```python
from build123d import *

# Parameters (mm, degrees)
BOSS_EXTRUDE1_DEPTH = 5.842
SKETCH2_R           = 3.175
CUT_EXTRUDE1_DEPTH  = 50.679572542


with BuildPart() as part:
    # Sketch1 → Boss-Extrude1 (new body)
    with BuildSketch(Plane(origin=(0, 0, 0), x_dir=(1, 0, 0), z_dir=(0, 1, 0))):
        Polygon((38.1, -25.5), (31.725545431, -25.5), (31.725545431, -31.342), (19.025545431, -31.342), (19.025545431, -25.5), (14.4526, -25.5), (14.4526, -19.15), (15.748, -19.15), (15.748, -15.975), (14.4526, -15.975), (14.4526, -11.403), (10.9474, -11.403), (10.9474, -15.975), (9.652, -15.975), (9.652, -19.15), (10.9474, -19.15), (10.9474, -25.5), (6.325545431, -25.5), (6.325545431, -31.342), (-6.374454569, -31.342), (-6.374454569, -25.5), (-10.996309138, -25.5), (-10.996309138, -19.15), (-9.700909138, -19.15), (-9.700909138, -15.975), (-10.996309138, -15.975), (-10.996309138, -11.403), (-14.501509138, -11.403), (-14.501509138, -15.975), (-15.796909138, -15.975), (-15.796909138, -19.15), (-14.501509138, -19.15), (-14.501509138, -25.5), (-19.074454569, -25.5), (-19.074454569, -31.342), (-31.774454569, -31.342), (-31.774454569, -25.5), (-38.1, -25.5), (-38.1, 25.5), (-31.774454569, 25.5), (-31.774454569, 31.342), (-19.074454569, 31.342), (-19.074454569, 25.5), (-14.501509138, 25.5), (-14.501509138, 19.15), (-15.796909138, 19.15), (-15.796909138, 15.975), (-14.501509138, 15.975), (-14.501509138, 11.403), (-10.996309138, 11.403), (-10.996309138, 15.975), (-9.700909138, 15.975), (-9.700909138, 19.15), (-10.996309138, 19.15), (-10.996309138, 25.5), (-6.374454569, 25.5), (-6.374454569, 31.342), (6.325545431, 31.342), (6.325545431, 25.5), (10.9474, 25.5), (10.9474, 19.15), (9.652, 19.15), (9.652, 15.975), (10.9474, 15.975), (10.9474, 11.403), (14.4526, 11.403), (14.4526, 15.975), (15.748, 15.975), (15.748, 19.15), (14.4526, 19.15), (14.4526, 25.5), (19.025545431, 25.5), (19.025545431, 31.342), (31.725545431, 31.342), (31.725545431, 25.5), (38.1, 25.5), align=None)
    extrude(amount=BOSS_EXTRUDE1_DEPTH)

    # Sketch2 → Cut-Extrude1 (cut, through all)
    with BuildSketch(Plane(origin=(0, 5.842, 0), x_dir=(1, 0, 0), z_dir=(0, 1, 0))):
        with Locations(Location((0, 0, 0), (0, 0, 270))):
            Circle(SKETCH2_R)
        with Locations(Location((25.4, 0, 0), (0, 0, 270))):
            Circle(SKETCH2_R)
        with Locations(Location((-25.448909138, 0, 0), (0, 0, 90))):
            Circle(SKETCH2_R)
    extrude(amount=-CUT_EXTRUDE1_DEPTH, mode=Mode.SUBTRACT)


solid = part.part
```
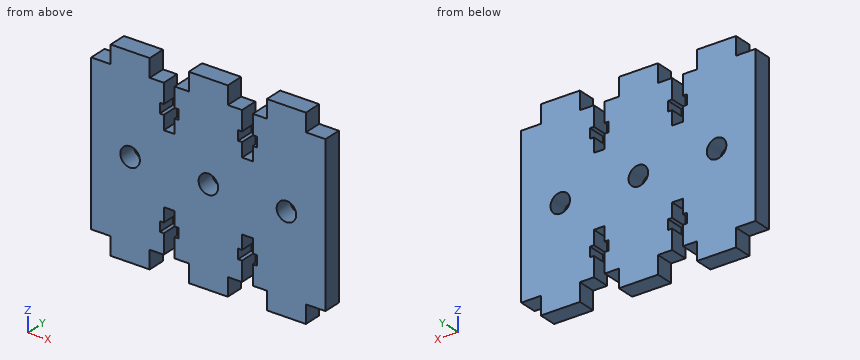
Verification items for the finished model (mm, model axes). Give positions to 0.01 mm unless a question says otherwise; leave off trailing zeros. Order: outer loops, then holes, each group sorted by start corner. A loop starts at its lowest first (then second) coordinate and runs counter-clockwise, first axis right, second up. Notation, with made-up numbers: M 12.5,-38 L 28.5,-38 A21 cw 28.5,-30 Z; hole C 89,20.5 d2. An arc over 180 degrees is marked long. Answer in a Markdown table with one row per item. Add a question column.
Item 1: Section check C-C, the plane z = 0. Enter the section's corners in (x, y) (3 decimals).
Item 2: Section check B-B, the plane z = -24. Enter the section's corners in (x, y), and give its area (3 significant figures).
Item 3: Scan lines: probe 1 along X at (y, z) = (4.7, 13); probe 2 along X at (y, z) = (3.05, 0) (3 decimals); probe 3 along X at (y, z) = (5.1, -19). Record each from-to range of solid material in increasing order. Write a range as from..to.
Item 4: Gauge pin test, flat ends, axial feed: pin 1 (3 mm diameter, centred on y = 2, z = -29.5, fed in from -X); pin 2 (1.1 mm diameter, centred on x = -13, y = 2.5, fed in from -Z); pin 3 (1.1 mm diameter, centred on x = -12, y = 1.5, fed in from +Z). Record the tip position at first contact, or that the pin passes through.
Item 5: Section check D-D, the plane x = -17. Enter the section's corners in (y, z), and give its area (3 significant figures).
Item 6: Section check A-A, the plane x = 25.4. Enter the section's corners in (y, z) (3 decimals).
Filled sheet:
| question | item | result |
|---|---|---|
| 1 | outline | M -38.1,0 L -28.624,0 L -28.624,5.842 L -38.1,5.842 Z; M -22.274,0 L -3.175,0 L -3.175,5.842 L -22.274,5.842 Z; M 3.175,0 L 22.225,0 L 22.225,5.842 L 3.175,5.842 Z; M 28.575,0 L 38.1,0 L 38.1,5.842 L 28.575,5.842 Z |
| 2 | outline | M -38.1,0 L -14.5,0 L -14.5,5.84 L -38.1,5.84 Z; M -11,0 L 10.95,0 L 10.95,5.84 L -11,5.84 Z; M 14.45,0 L 38.1,0 L 38.1,5.84 L 14.45,5.84 Z |
| 2 | area | 404 mm^2 |
| 3 | probe 1 | x = -38.1..-14.5, -11..10.95, 14.45..38.1 |
| 3 | probe 2 | x = -38.1..-28.624, -22.274..-3.175, 3.175..22.225, 28.575..38.1 |
| 3 | probe 3 | x = -38.1..-15.8, -9.7..9.65, 15.75..38.1 |
| 4 | pin 1 | stops at x = -31.77 |
| 4 | pin 2 | stops at z = -11.4 |
| 4 | pin 3 | stops at z = 11.4 |
| 5 | outline | M 0,-25.5 L 5.84,-25.5 L 5.84,25.5 L 0,25.5 Z |
| 5 | area | 298 mm^2 |
| 6 | outline | M 0,-31.342 L 5.842,-31.342 L 5.842,-3.175 L 0,-3.175 Z; M 0,3.175 L 5.842,3.175 L 5.842,31.342 L 0,31.342 Z |
